Can you work these out from the model? Positions are in its coordinate system, mm. Coordinates: 2 decimals unless noted, no trailing zeros. Order: outer loops, then holes, each group sorted by start corner. A loop starts at its lowest first (then second) coordinate and runs counter-clockwise, first axis right, second up. Notation, with made-up numbers: (62.25, 4) -> (97.25, 4) arc R24 ccw to (97.25, 25) -> close; hole circle Ø3 at (-30, 45). An arc over 180 degrees is marked (long way). Return JSON: item names as keys, results as strings. Group by question number.
1) If we section it at B-B, the plane z = 13: Please give me the cut outline in (x, y), then the cut area to 3 significant figures.
2) If we section it at A-A, the plane y = 34.5: Please give me the cut outline in (x, z).
3) For pin 1 (10 mm diameter, centred on y = 58, z = 16.5, fed in from -X); pin 2 (5 mm diameter, centred on y = 38, z = 13, fed in from -X), each with a flat end and sliding along its axis, tell me the tip position at first contact or that it passes through.
4) If I drill on probe 1 along Y at (x, z) = (862, 1.5); probe 2 along X at (y, z) = (91, 10.5); probe 3 along X at (y, z) = (21.5, 2.5), over which ranges is the centre line in solid material (lowest first)? Write a range as from..to.
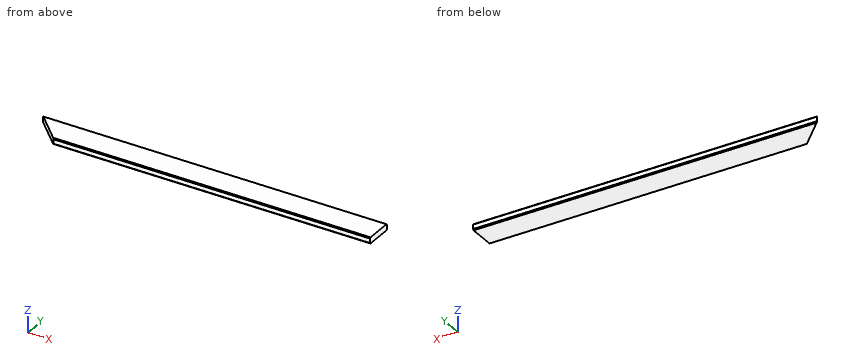
from build123d import *

# Parameters (mm, degrees)
ESQUISSE1_W                  = 1950
ESQUISSE1_H                  = 100
BOSS_EXTRU_1_DEPTH           = 22
ENL_V_MAT_EXTRU_1_DEPTH      = 1953.686354743
ENL_V_MAT_EXTRU_1_DEPTH_BACK = 1953.686354743
CHANFREIN1_SIZE              = 3


with BuildPart() as part:
    # Esquisse1 → Boss.-Extru.1 (new body)
    with BuildSketch(Plane.XY):
        with Locations((975, 50)):
            Rectangle(ESQUISSE1_W, ESQUISSE1_H)
    extrude(amount=BOSS_EXTRU_1_DEPTH)

    # Esquisse2 → Enlèv. mat.-Extru.1 (cut, two sides: drawn at the far end of the back side and taken through both)
    with BuildSketch(Plane(origin=(0, 0, 0), x_dir=(-1, 0, 0), z_dir=(0, 0, -1)).offset(-ENL_V_MAT_EXTRU_1_DEPTH_BACK)):
        Polygon((0, 0), (-800, 0), (-700, 100), (0, 100), align=None)
    extrude(amount=ENL_V_MAT_EXTRU_1_DEPTH + ENL_V_MAT_EXTRU_1_DEPTH_BACK, mode=Mode.SUBTRACT)

    # Chanfrein1
    chanfrein1_edges = [part.edges().sort_by_distance(p)[0] for p in [
        (1325, 100, 22),
        (1375, 0, 0),
        (1375, 0, 22),
        (1325, 100, 0),
    ]]
    chamfer(chanfrein1_edges, length=CHANFREIN1_SIZE)


solid = part.part
Result sheet:
{
 "1": {"outline": "(700, 100) -> (800, 0) -> (1950, 0) -> (1950, 100) -> close", "area": "120,000 mm2"},
 "2": {"outline": "(765.5, 0) -> (1950, 0) -> (1950, 22) -> (765.5, 22) -> close"},
 "3": {"pin 1": "stops at x = 737", "pin 2": "stops at x = 759.5"},
 "4": {"probe 1": "y = 1.5..98.5", "probe 2": "x = 709..1950", "probe 3": "x = 778.5..1950"}
}
